```python
from build123d import *

# Parameters (mm, degrees)
SKETCH1_R                    = 20
SKETCH1_R_2                  = 3.5
BOSS_EXTRUDE1_DEPTH          = 5
BOSS_EXTRUDE2_DEPTH          = 12.7
BOSS_EXTRUDE2_DEPTH_BACK     = 12.7
SKETCH3_R                    = 5.75
SKETCH3_R_2                  = 3.5
F_4_0_4_DIAMETER_HOLE1_D     = 4
F_4_0_4_DIAMETER_HOLE1_DEPTH = 15
F_4_0_4_DIAMETER_HOLE1_TIP   = 1.201721238


with BuildPart() as part:
    # Sketch1 → Boss-Extrude1 (new body)
    with BuildSketch(Plane(origin=(0, 0, 0), x_dir=(0, 0, -1), z_dir=(1, 0, 0))):
        Circle(SKETCH1_R)
        Circle(SKETCH1_R_2, mode=Mode.SUBTRACT)
    extrude(amount=BOSS_EXTRUDE1_DEPTH)

    # Sketch3 → Boss-Extrude2 (add, two sides: drawn at the far end of the back side and taken through both)
    with BuildSketch(Plane.ZY.offset(-BOSS_EXTRUDE2_DEPTH_BACK)):
        Circle(SKETCH3_R)
        Circle(SKETCH3_R_2, mode=Mode.SUBTRACT)
    extrude(amount=BOSS_EXTRUDE2_DEPTH + BOSS_EXTRUDE2_DEPTH_BACK)

    # Ø4.0 (4) Diameter Hole1
    with Locations(Plane(origin=(5, 0, 0), x_dir=(0, 0, -1), z_dir=(1, 0, 0))):
        with Locations((12.5, 0), (0, -12.5), (-12.5, 0), (0, 12.5)):
            Hole(F_4_0_4_DIAMETER_HOLE1_D / 2, depth=F_4_0_4_DIAMETER_HOLE1_DEPTH)
            with Locations((0, 0, -(F_4_0_4_DIAMETER_HOLE1_DEPTH + F_4_0_4_DIAMETER_HOLE1_TIP / 2))):  # 118° drill point
                Cone(0, F_4_0_4_DIAMETER_HOLE1_D / 2, F_4_0_4_DIAMETER_HOLE1_TIP, mode=Mode.SUBTRACT)


solid = part.part
```
Work out the finished part from the listing and answer in its coordinate system (mm). A direction names the side the tool comes from. Round coordinates to 2 decimals unless told otherwise and drop trailing zeros. Loops run counter-clockwise (first coordinate to the right, second up) from the corner with the lowest first, then second, coordinate; pieces in that order, holes last.
(1) The part is cut by section A-A, the plane z = 0. Give the vertices of the cut face in (x, y).
Computed values:
outline: (-12.7, -5.75) - (0, -5.75) - (0, -10.5) - (5, -10.5) - (5, -5.75) - (12.7, -5.75) - (12.7, -3.5) - (-12.7, -3.5) - close; (-12.7, 3.5) - (12.7, 3.5) - (12.7, 5.75) - (5, 5.75) - (5, 10.5) - (0, 10.5) - (0, 5.75) - (-12.7, 5.75) - close; (0, -20) - (5, -20) - (5, -14.5) - (0, -14.5) - close; (0, 14.5) - (5, 14.5) - (5, 20) - (0, 20) - close
(2) The part is cut by section C-C, the plane x = -8.25. Give the vertices of the cut face in (y, z).
Computed values:
outline: circle Ø11.5 at (0, 0); hole circle Ø7 at (0, 0)
(3) The mould has two halves that part along Y. Classify faces 3 (the cylindrical face through (-6.26, 5.7, -0.75)), 4 (the cylindrical face through (2.5, -1.2, -14.1)), 5 (the flat face through (0, -4.2, -4.2)): pulls with the +Y half, pulls with the -Y half, needs draft (parallel to the pull), parting line crosses it, or undercut.
Computed values:
face 3: parting line crosses it
face 4: undercut
face 5: needs draft
(4) For faces 1 (the cylindrical face through (2.465, 14.483, -0.26)), 2 (the cylindrical face through (8.9, 5.7, -0.75)), determine the directions among +Z, -Z, +X, -X, +Y, -Y from which every point of the face is accessible in a straight line to the end or side of a thin tool.
Computed values:
face 1: +X, -X
face 2: +X
(5) Each of these flat-tipped pins is pushed along its axis until it touches: P1, Ø1.5, axis at x = 1, z = 12.5, coming from the +Y side; P2, Ø12, axis at x = 5, z = -3.5, coming from the -Y side; P3, Ø2, axis at x = 5, y = -3, coming from the -Z side; P4, Ø6, axis at y = -7, z = -4.5, coming from the -X side. Where does it stop, or does it pass through?
Computed values:
P1: stops at y = 16.18
P2: stops at y = -20
P3: stops at z = -19.9
P4: stops at x = -12.7
(6) The part is cut by section B-B, the plane y = 12.5. Give the vertices of the cut face in (x, z), and give its area (3 significant figures).
Computed values:
outline: (0, -15.61) - (5, -15.61) - (5, -2) - (0, -2) - close; (0, 2) - (5, 2) - (5, 15.61) - (0, 15.61) - close
area: 136 mm2
(7) Find the intervals of material crossed by L1, parallel to Y at x = 8.5, z = 0; L2, parallel to Y at x = 1.4, z = -12.5, in increasing order.
Computed values:
L1: y = -5.75 to -3.5, 3.5 to 5.75
L2: y = -15.61 to -2, 2 to 15.61
